The model under review builds one solid part; all positions refer to its coordinate system, in mm. Coordinates: 2 decimals unless noted, no trailing zeros. Order: outer loops, then holes, each group sorted by start corner. A loop starts at its lowest first (then second) coordinate and runs counter-clockwise, first axis right, second up. Notation, with made-up numbers: M 9.25,10.5 L 37.25,10.5 A10 cw 37.25,24.5 Z; hole C -7,-2 d10. An arc over 180 degrees is marked long. Write each question's results on one line, items separated by ' | '.
from build123d import *

# Parameters (mm, degrees)
F1_W     = 65
F1_H     = 40
F1_R     = 1.5
F1_W_2   = 8
F1_H_2   = 3
F2_DEPTH = 3
F3_R     = 5
F5_D     = 4.4


with BuildPart() as f2:
    # F1 (on Top) → F2 (new body)
    with BuildSketch(Plane.XY):
        Rectangle(F1_W, F1_H)
        with Locations((-24.5, -14)):
            Circle(F1_R, mode=Mode.SUBTRACT)
        with Locations((-14, -14)):
            Rectangle(F1_W_2, F1_H_2, mode=Mode.SUBTRACT)
        with Locations((14, -14)):
            Rectangle(F1_W_2, F1_H_2, mode=Mode.SUBTRACT)
        with Locations((24.5, -14)):
            Circle(F1_R, mode=Mode.SUBTRACT)
        with Locations((-24.5, 14)):
            Circle(F1_R, mode=Mode.SUBTRACT)
        with Locations((-14, 14)):
            Rectangle(F1_W_2, F1_H_2, mode=Mode.SUBTRACT)
        with Locations((14, 14)):
            Rectangle(F1_W_2, F1_H_2, mode=Mode.SUBTRACT)
        with Locations((24.5, 14)):
            Circle(F1_R, mode=Mode.SUBTRACT)
    extrude(amount=F2_DEPTH)

    # F3
    f3_edges = [f2.edges().sort_by_distance(p)[0] for p in [
        (-32.5, -20, 1.5),
        (-32.5, 20, 1.5),
        (32.5, -20, 1.5),
        (32.5, 20, 1.5),
    ]]
    fillet(f3_edges, radius=F3_R)

    # F5 (through all)
    with Locations(Plane.XY.offset(3)):
        with Locations((-12.5, 6.125), (-12.5, -6.375), (12.5, 6.125), (12.5, -6.375)):
            Hole(F5_D / 2)


solid = f2.part
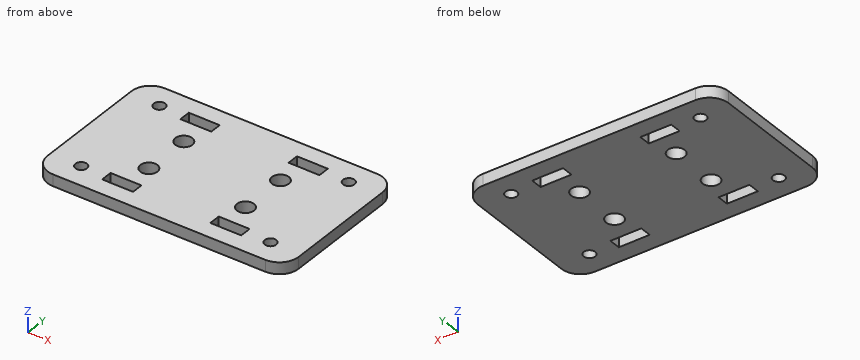
1) Take a section at D-D on y = -14. State the section outline as (x, z) points, plus the area to 3 significant figures.
Solutions:
outline: M -32.5,0 L -26,0 L -26,3 L -32.5,3 Z; M -23,0 L -18,0 L -18,3 L -23,3 Z; M -10,0 L 10,0 L 10,3 L -10,3 Z; M 18,0 L 23,0 L 23,3 L 18,3 Z; M 26,0 L 32.5,0 L 32.5,3 L 26,3 Z | area: 129 mm2
2) Take a section at A-A on x = 24.5. State the section outline as (y, z) points.
Solutions:
outline: M -20,0 L -15.5,0 L -15.5,3 L -20,3 Z; M -12.5,0 L 12.5,0 L 12.5,3 L -12.5,3 Z; M 15.5,0 L 20,0 L 20,3 L 15.5,3 Z
3) To check wall thickness, follow line 1 along Y through (x, z) = (-24.5, 0.8); line 2 along Y through (x, z) = (12.5, 1) (3 decimals); line 3 along X through (y, z) = (-15, 1.5). State the ranges of each line that lie inside material, in increasing order.
Solutions:
line 1: -20 to -15.5, -12.5 to 12.5, 15.5 to 20 | line 2: -20 to -15.5, -12.5 to -8.575, -4.175 to 3.925, 8.325 to 12.5, 15.5 to 20 | line 3: -32.5 to -25.62, -23.38 to -18, -10 to 10, 18 to 23.38, 25.62 to 32.5
4) Take a section at B-B on y = -5.5. State the section outline as (x, z) points, plus the area to 3 significant figures.
Solutions:
outline: M -32.5,0 L -14.52,0 L -14.52,3 L -32.5,3 Z; M -10.48,0 L 10.48,0 L 10.48,3 L -10.48,3 Z; M 14.52,0 L 32.5,0 L 32.5,3 L 14.52,3 Z | area: 171 mm2
5) For pin 1 (12 mm diameter, centred on x = -15, y = 11.5, fed in from -Z), flat-tipped, find the tip position at first contact; note if it passes through.
Solutions:
pin 1: z = 0
6) Take a section at C-C on x = -12.5. State the section outline as (y, z) points (3 decimals).
Solutions:
outline: M -20,0 L -15.5,0 L -15.5,3 L -20,3 Z; M -12.5,0 L -8.575,0 L -8.575,3 L -12.5,3 Z; M -4.175,0 L 3.925,0 L 3.925,3 L -4.175,3 Z; M 8.325,0 L 12.5,0 L 12.5,3 L 8.325,3 Z; M 15.5,0 L 20,0 L 20,3 L 15.5,3 Z
